Here's how the part is built. I have some questions about the finished solid (model axes, mm). Round coordinates to 2 decimals unless told otherwise and drop trailing zeros. Write each loop counter-clockwise with the first axis right and the second up, starting at its lowest first coordinate (ties: lowest second). Pieces come first, ordered by that corner, then holes. Notation, with made-up numbers: (25.5, -17) -> (74.5, -17) arc R37 cw to (74.5, 21) -> close; hole circle Ø1 at (-37, -35). An arc over 180 degrees is marked (long way). Answer as CSV lines item,"result".
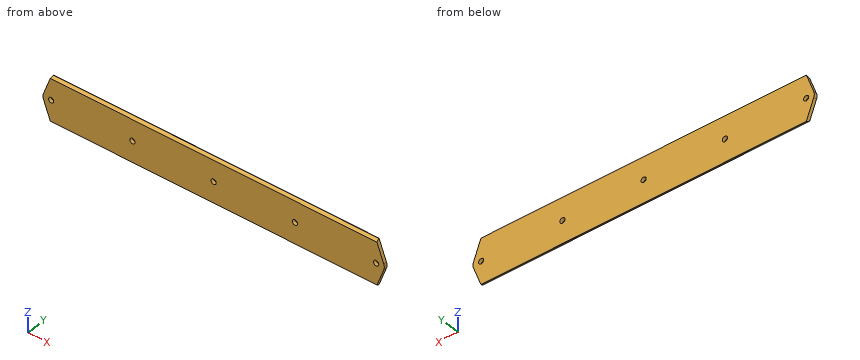
from build123d import *

# Parameters (mm, degrees)
SKETCH_1_R               = 1.6
EXTRUDE_1_DEPTH          = 2
CUT_EXTRUDE_1_DEPTH      = 5
CUT_EXTRUDE_1_DEPTH_BACK = 210
CHAMFER_2_SIZE           = 0.2
CHAMFER_2_SIZE_2         = 0.1


with BuildPart() as part:
    # Эскиз1 → Бобышка-Вытянуть1 (new body)
    with BuildSketch(Plane(origin=(0, 0, 0), x_dir=(1, 0, 0), z_dir=(0, 1, 0))):
        with BuildLine():
            Line((-125, 14), (75, 14))
            Line((75, 14), (79.670248868, 1.785714286))
            ThreePointArc((79.670248868, 1.785714286), (80, 0), (79.670248868, -1.785714286))
            Line((79.670248868, -1.785714286), (75, -14))
            Line((75, -14), (-75, -14))
            Line((-75, -14), (-125, -14))
            Line((-125, -14), (-129.670248868, -1.785714286))
            ThreePointArc((-129.670248868, -1.785714286), (-130, 0), (-129.670248868, 1.785714286))
            Line((-129.670248868, 1.785714286), (-125, 14))
        make_face()
        with Locations(Location((-75, 0, 0), (0, 0, 270))):
            Circle(SKETCH_1_R, mode=Mode.SUBTRACT)
        with Locations(Location((75, 0, 0), (0, 0, 270))):
            Circle(SKETCH_1_R, mode=Mode.SUBTRACT)
        with Locations(Location((-25, 0, 0), (0, 0, 270))):
            Circle(SKETCH_1_R, mode=Mode.SUBTRACT)
        with Locations(Location((25, 0, 0), (0, 0, 270))):
            Circle(SKETCH_1_R, mode=Mode.SUBTRACT)
        with Locations(Location((-125, 0, 0), (0, 0, 270))):
            Circle(SKETCH_1_R, mode=Mode.SUBTRACT)
    extrude(amount=EXTRUDE_1_DEPTH)

    # Эскиз4 → Вырез-Вытянуть1 (cut, two sides: drawn at the far end of the back side and taken through both)
    with BuildSketch(Plane.ZY.offset(125).offset(-CUT_EXTRUDE_1_DEPTH_BACK)):
        Polygon((-14, 2), (-14, 0), (-12.645299462, 0), (-13.8, 2), align=None)
        Polygon((14, 2), (14, 0), (12.645299462, 0), (13.8, 2), align=None)
    extrude(amount=CUT_EXTRUDE_1_DEPTH + CUT_EXTRUDE_1_DEPTH_BACK, mode=Mode.SUBTRACT)

    # Фаска2
    # the kernel refuses this chamfer: 0.2, 0.1 mm, written as the material it takes off along each edge
    with BuildSketch(Plane(origin=(-125.593889062, 2, -13.8), x_dir=(0, -0.875527030904719, 0.48316914031751595), z_dir=(1, 0, 0))) as chamfer_2_piece_1:
        Polygon((CHAMFER_2_SIZE * 0.999813220622, -CHAMFER_2_SIZE * 0.0193267656127), (CHAMFER_2_SIZE_2 * 0.483169140318, -CHAMFER_2_SIZE_2 * 0.875527030905), (0, 0), align=None)
    extrude(amount=201.187778124, mode=Mode.SUBTRACT)
    with BuildSketch(Plane(origin=(75.593889062, 2, 13.8), x_dir=(1.1200704684646426e-15, 0.07974522228289034, -0.996815278536125), z_dir=(-1, 0, 0))) as chamfer_2_piece_2:
        Polygon((CHAMFER_2_SIZE_2 * 0.996815278536, CHAMFER_2_SIZE_2 * 0.0797452222829), (CHAMFER_2_SIZE * 0.429346250941, CHAMFER_2_SIZE * 0.903139965234), (0, 0), align=None)
    extrude(amount=201.187778124, mode=Mode.SUBTRACT)


solid = part.part
Item 1: I need wall thicknesses on L1, parallel to X at y = 1.5, z = 0; L2, parallel to X at y = 1.05, z = 1.25; L3, parallel to Z at x = -125, y = 1.55. Which ranges of each line are inside material? Lowest first, please.
Results found:
L1,"x = -130 to -126.6, -123.4 to -76.6, -73.4 to -26.6, -23.4 to 23.4, 26.6 to 73.4, 76.6 to 80"
L2,"x = -129.84 to -126, -124 to -76, -74 to -26, -24 to 24, 26 to 74, 76 to 79.84"
L3,"z = -13.54 to -1.6, 1.6 to 13.54"
Item 2: Suppose I cut it at C-C, the plane z = 5.5. List the corners of the cut face in (x, y) for me, then the cut area to 3 significant figures.
Results found:
outline,"(-128.25, 0) -> (78.25, 0) -> (78.25, 2) -> (-128.25, 2) -> close"
area,"413 mm²"
Item 3: Suppose I cut it at B-B, the plane x = -71.5. List the corners of the cut face in (y, z) for me.
Results found:
outline,"(0, -12.65) -> (1.83, -13.7) -> (2, -13.7) -> (2, 13.7) -> (1.83, 13.7) -> (0, 12.65) -> close"
Item 4: Suppose I cut it at A-A, the plane y = 0.55. List the corners of the cut face in (x, z) for me, then the cut area to 3 significant figures.
Results found:
outline,"(-129.67, -1.79) -> (-125.4, -12.96) -> (75.4, -12.96) -> (79.67, -1.79) arc R5 ccw to (79.67, 1.79) -> (75.4, 12.96) -> (-125.4, 12.96) -> (-129.67, 1.79) arc R5 ccw to start; hole circle Ø3.2 at (-125, 0); hole circle Ø3.2 at (-75, 0); hole circle Ø3.2 at (-25, 0); hole circle Ø3.2 at (25, 0); hole circle Ø3.2 at (75, 0)"
area,"5,290 mm²"
